Autodesk Inventor part; units mm, degrees
ref_plane "YZ Plane" through (0, 0, 0) normal (1, 0, 0) x (0, 1, 0)
ref_plane "XZ Plane" through (0, 0, 0) normal (0, 1, 0) x (-1, 0, 0)
ref_plane "XY Plane" through (0, 0, 0) normal (0, 0, 1) x (1, 0, 0)
sketch "Sketch1" plane through (0, 0, 0) normal (0, 0, 1) x (1, 0, 0)
  circle A0 centre (0, 0) radius 5
  circle A1 centre (0, 0) radius 9
  dimension "d0" = 10
  dimension "d1" = 18
extrude "Extrusion1" add sketch "Sketch1" along normal blind 7
thread "Thread1"
sketch "Sketch13" plane through (0, 0, 7) normal (0, 0, 1) x (1, 0, 0)
  line L0 (-15.4051, -11.6713) -> (15.4051, -11.6713)
  line L1 (15.4051, -11.6713) -> (15.4051, 11.6713)
  line L2 (15.4051, 11.6713) -> (-15.4051, 11.6713)
  line L3 (-15.4051, 11.6713) -> (-15.4051, -11.6713)
  line L4 (-15.4051, -11.6713) -> (15.4051, 11.6713) construction
  line L5 (15.4051, -11.6713) -> (-15.4051, 11.6713) construction
  point P0 (0, 0)
  dimension "d50" = 30.8102
  dimension "d51" = 23.3426
extrude "Extrusion13" add sketch "Sketch13" along normal blind 10
sketch "Sketch14" plane through (0, 0, 17) normal (0, 0, 1) x (1, 0, 0)
  line L0 (-12.5334, -9) -> (12.5334, -9)
  line L1 (12.5334, -9) -> (12.5334, 9)
  line L2 (12.5334, 9) -> (-12.5334, 9)
  line L3 (-12.5334, 9) -> (-12.5334, -9)
  line L4 (-12.5334, -9) -> (12.5334, 9) construction
  line L5 (12.5334, -9) -> (-12.5334, 9) construction
  point P0 (0, 0)
extrude "Extrusion14" cut sketch "Sketch14" against normal blind 7
sketch "Sketch15" plane through (0, 0, 7) normal (0, 0, -1) x (-1, 0, 0)
  circle A0 centre (0, 0) radius 5
extrude "Extrusion15" cut sketch "Sketch15" against normal blind 7
properties part number "Newairtempguy"
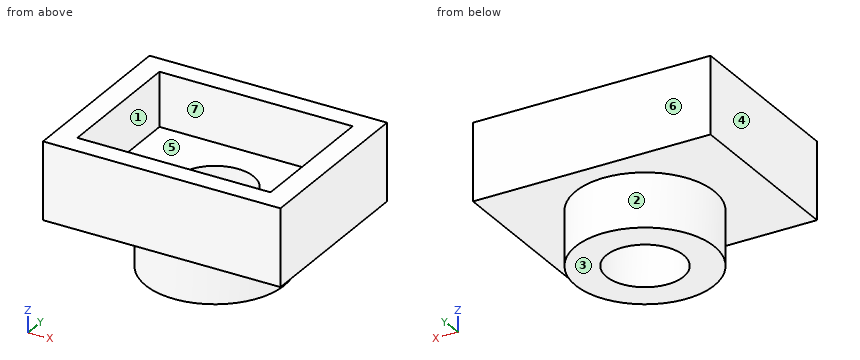
Here's how the part is built. I have some questions about the finished solid (model axes, mm). Face numbers are marked on the shaded views. A direction names the side the tool comes from. Round coordinates to 2 decimals unless told otherwise and drop trailing zeros. Order: outer loops, then holes, each group sorted by start corner. A loop starts at its lowest first (then second) coordinate and runs counter-clockwise, first axis right, second up. Notation, with made-up numbers: M -4.5,34.25 L 40.5,34.25 A10 cw 40.5,47.25 Z; hole C 5,-16.5 d3. An arc over 180 degrees is marked long. Return JSON: item names as keys, results as strings. Group by question number.
1. Please list where these lines run through material, in increasing order: probe 1 along Y at (x, z) = (0, 8.95); probe 2 along X at (y, z) = (0, 8.6); probe 3 along Z at (x, y) = (3.5, 6.75).
2. On a 3-axis mill with a long thin cutter (end or side, diameter ignored), from which of +Z, -Z, +X, -X, +Y, -Y can I reach the whole of each face in a straight line? I mean the marked faces 1, 2 and 3. Say none if no direction works.
3. If we mould it in two halves opening along Y, with no side actions, what happens to the marked faces 4, 5, 6 and 7? For each: pulls with the +Y half, pulls with the -Y half, needs draft (parallel to the pull), parting line crosses it, or undercut.
4. If we section it at C-C on z = 13.25: List the corners of the cut face in (x, y) for me.
5. If we section it at A-A on x = 0: List the corners of the cut face in (y, z) for me, then the cut area to 3 significant figures.
6. I'm going to push flat-ended pins straight in: pin 1 Ø2 at (x, y) = (2.5, 6) entering from +Z; pin 2 Ø3 at (x, y) = (-10.5, 5) entering from -Z; pin 3 Ø1.5 at (y, z) = (0, 4) entering from -X. Where does each tip first touch, or does it pass through?
7. If we section it at B-B on y = 0: List the corners of the cut face in (x, z) for me.
8. If we section it at D-D on x = 10: List the corners of the cut face in (y, z) for me.
Reply:
{
 "1": {"probe 1": "-11.67 to -5, 5 to 11.67", "probe 2": "-15.41 to -5, 5 to 15.41", "probe 3": "0 to 10"},
 "2": {"face 1": "+Z", "face 2": "-Z", "face 3": "-Z, +X, -X, +Y, -Y"},
 "3": {"face 4": "needs draft", "face 5": "undercut", "face 6": "pulls with the +Y half", "face 7": "undercut"},
 "4": {"outline": "M -15.41,-11.67 L 15.41,-11.67 L 15.41,11.67 L -15.41,11.67 Z; hole M -12.53,-9 L 12.53,-9 L 12.53,9 L -12.53,9 Z"},
 "5": {"outline": "M -11.67,7 L -9,7 L -9,0 L -5,0 L -5,10 L -9,10 L -9,17 L -11.67,17 Z; M 5,0 L 9,0 L 9,7 L 11.67,7 L 11.67,17 L 9,17 L 9,10 L 5,10 Z", "area": "133 mm^2"},
 "6": {"pin 1": "z = 10", "pin 2": "z = 7", "pin 3": "x = -9"},
 "7": {"outline": "M -15.41,7 L -9,7 L -9,0 L -5,0 L -5,10 L -12.53,10 L -12.53,17 L -15.41,17 Z; M 5,0 L 9,0 L 9,7 L 15.41,7 L 15.41,17 L 12.53,17 L 12.53,10 L 5,10 Z"},
 "8": {"outline": "M -11.67,7 L 11.67,7 L 11.67,17 L 9,17 L 9,10 L -9,10 L -9,17 L -11.67,17 Z"}
}
